```python
from build123d import *

# Parameters (mm, degrees)
SKETCH_4_R               = 10
EXTRUDE_2_DEPTH          = 2.5
SKETCH_6_R               = 1.5
CUT_EXTRUDE_9_DEPTH      = 2.5
SKETCH_7_R               = 4.4
EXTRUDE_3_DEPTH          = 2
SKETCH_8_R               = 3
CUT_EXTRUDE_10_DEPTH     = 3
EXTRUDE_5_DEPTH          = 2
PATTERN_CIRCULAR_1_COUNT = 24


with BuildPart() as part:
    # Sketch 4 → Extrude 2 (new body)
    with BuildSketch(Plane(origin=(0, 0, 0), x_dir=(1, 0, 0), z_dir=(0, 1, 0))):
        Circle(SKETCH_4_R)
    extrude(amount=EXTRUDE_2_DEPTH)

    # Sketch 6 → Cut-Extrude 9 (cut)
    with BuildSketch(Plane(origin=(0, 2.5, 0), x_dir=(1, 0, 0), z_dir=(0, 1, 0))):
        with Locations((0, 7)):
            Circle(SKETCH_6_R)
        Circle(SKETCH_6_R)
        with Locations((7, 0)):
            Circle(SKETCH_6_R)
        with Locations((-7, 0)):
            Circle(SKETCH_6_R)
        with Locations((0, -7)):
            Circle(SKETCH_6_R)
    extrude(amount=-CUT_EXTRUDE_9_DEPTH, mode=Mode.SUBTRACT)

    # Sketch 7 → Extrude 3 (add)
    with BuildSketch(Plane(origin=(0, 2.5, 0), x_dir=(1, 0, 0), z_dir=(0, 1, 0))):
        Circle(SKETCH_7_R)
    extrude(amount=EXTRUDE_3_DEPTH)

    # Sketch 8 → Cut-Extrude 10 (cut)
    with BuildSketch(Plane(origin=(0, 4.5, 0), x_dir=(1, 0, 0), z_dir=(0, 1, 0))):
        Circle(SKETCH_8_R)
    extrude(amount=-CUT_EXTRUDE_10_DEPTH, mode=Mode.SUBTRACT)

    # Sketch 14 → Extrude 5 (add)
    with BuildSketch(Plane(origin=(0, 4.5, 0), x_dir=(1, 0, 0), z_dir=(0, 1, 0))):
        with BuildLine():
            Line((2.976910005, -0.371492698), (2.495792863, -0.23538136))
            Line((2.495792863, -0.23538136), (2.495792863, 0.032272898))
            Line((2.495792863, 0.032272898), (2.995792863, 0.158824181))
            ThreePointArc((2.995792863, 0.158824181), (2.998100046, -0.106752588), (2.976910005, -0.371492698))
        make_face()
    extrude_5 = extrude(amount=-EXTRUDE_5_DEPTH)

    # Pattern Circular 1: Extrude 5 ×24 about axis
    pattern_circular_1_axis = Axis((0, 0, 0), (0, 1, 0))
    for i in range(1, PATTERN_CIRCULAR_1_COUNT):
        add(extrude_5.rotate(pattern_circular_1_axis, i * 360 / PATTERN_CIRCULAR_1_COUNT))


solid = part.part
```
Read the model definition and answer for the solid it produces. Units are mm, in the model's axes. A direction names the side the tool comes from. Coordinates: 2 decimals unless noted, no trailing zeros. Write each loop counter-clockwise with the first axis right and the second up, starting at its lowest first coordinate (ties: lowest second). Pieces come first, ordered by that corner, then holes. Notation, with made-up numbers: (12.25, -34) -> (41.25, -34) arc R32 cw to (41.25, 1) -> close; hole circle Ø3 at (57, 40). An arc over 180 degrees is marked (long way). Return JSON: item names as keys, results as strings.
1. A cutting plane is placed at C-C (y = 1.05). Determine the outline of the cut face in (x, z), and give its area (3 significant figures).
Found:
{"outline": "circle Ø20 at (0, 0); hole circle Ø3 at (-7, 0); hole circle Ø3 at (0, -7); hole circle Ø3 at (0, 0); hole circle Ø3 at (0, 7); hole circle Ø3 at (7, 0)", "area": "279 mm2"}
2. This flat-tipped pin is pushed along its axis until it touches: P1, Ø2.5, axis at x = 0, z = 0, coming from the +Y side. Where does it stop, or does it pass through?
Found:
{"P1": "through"}
3. A tool of negligible diameter and unlimited length cuts with its end or side. For faces 5 (the face through (5.5, 1.27, -0.07)), 6 (the face through (4.3, 2.5, 2.1)), 7 (the face through (2.77, 2.35, 1.15)), from which of +Z, -Z, +X, -X, +Y, -Y can it reach the whole face along a straight path? Write none if from no direction.
Found:
{"face 5": "+Y, -Y", "face 6": "+Y", "face 7": "none"}
4. Determine the mould class of faces 1 (the face through (4.197, 3.486, -1.322)), 2 (the face through (1.3, 1.5, 1.3)), 3 (the face through (-1.5, 0.76, -0.07)), 4 (the face through (0, 4.5, 3)) for opening direction Z: pulls with the +Z half, pulls with the -Z half, needs draft (parallel to the pull), parting line crosses it, or undercut.
Found:
{"face 1": "parting line crosses it", "face 2": "undercut", "face 3": "undercut", "face 4": "needs draft"}
5. A cutting plane is placed at A-A (x = -7.25). Determine the outline of the cut face in (y, z).
Found:
{"outline": "(0, -6.89) -> (2.5, -6.89) -> (2.5, -1.48) -> (0, -1.48) -> close; (0, 1.48) -> (2.5, 1.48) -> (2.5, 6.89) -> (0, 6.89) -> close"}
6. A cutting plane is placed at B-B (z = 7). Determine the outline of the cut face in (x, y).
Found:
{"outline": "(-7.14, 0) -> (-1.5, 0) -> (-1.5, 2.5) -> (-7.14, 2.5) -> close; (1.5, 0) -> (7.14, 0) -> (7.14, 2.5) -> (1.5, 2.5) -> close"}
7. Find the intervals of material crossed by line 1 along Z through (x, y) = (0, 1.2); line 2 along Z through (x, y) = (0, 2.7), in increasing order. Write a range as from..to.
Found:
{"line 1": "-10..-8.5, -5.5..-1.5, 1.5..5.5, 8.5..10", "line 2": "-4.4..-2.5, 2.5..4.4"}
8. A cutting plane is placed at D-D (x = 3.25). Determine the outline of the cut face in (y, z), and give its area (4 significant figures).
Found:
{"outline": "(0, -9.46) -> (2.5, -9.46) -> (2.5, -2.97) -> (4.5, -2.97) -> (4.5, 2.97) -> (2.5, 2.97) -> (2.5, 9.46) -> (0, 9.46) -> close", "area": "59.15 mm2"}
